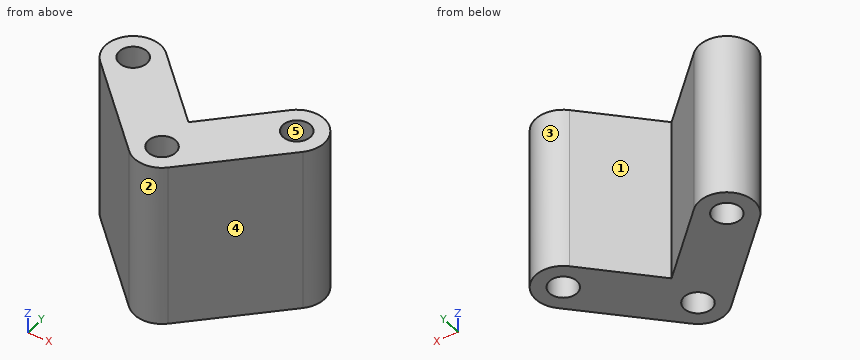
```python
from build123d import *

# Parameters (mm, degrees)
F0_R     = 12.5
F1_DEPTH = 150
F3_DEPTH = 50


# Not quite as in the source:
# - the program builds the solid bodies; features that only make, move or delete a surface that nothing else refers to are left out


with BuildPart() as f1:
    # F0 (on Top) → F1 (new body)
    with BuildSketch(Plane.XY):
        with BuildLine():
            Line((8.6845052377, -18.7444362128), (-50.6748429861, 39.3975202147))
            ThreePointArc((-50.6748429861, 39.3975202147), (-86.0282846169, 39.0312350068), (-85.661999409, 3.6777933759))
            Line((-85.661999409, 3.6777933759), (-9.0315715293, -71.3810327757))
            ThreePointArc((-9.0315715293, -71.3810327757), (8.4718011348, -78.5211674377), (25.9695737293, -71.3673200922))
            Line((25.9695737293, -71.3673200922), (98.7170861934, 0))
            ThreePointArc((98.7170861934, 0), (99.0182133881, 35.3918171352), (63.6258335307, 35.6173071466))
            Line((63.6258335307, 35.6173071466), (8.6845052377, -18.7444362128))
        make_face()
        with Locations((8.4620066821, -53.5211693563)):
            Circle(F0_R, mode=Mode.SUBTRACT)
        with Locations((-68.1684211975, 21.5376567953)):
            Circle(F0_R, mode=Mode.SUBTRACT)
        with Locations((81.2095191462, 17.8461507359)):
            Circle(F0_R, mode=Mode.SUBTRACT)
    extrude(amount=F1_DEPTH)

    # F0 (on Top) → F3 (join)
    with BuildSketch(Plane.XY):
        with BuildLine():
            Line((8.6845052377, -18.7444362128), (-50.6748429861, 39.3975202147))
            ThreePointArc((-50.6748429861, 39.3975202147), (-86.0282846169, 39.0312350068), (-85.661999409, 3.6777933759))
            Line((-85.661999409, 3.6777933759), (-9.0315715293, -71.3810327757))
            ThreePointArc((-9.0315715293, -71.3810327757), (8.4718011348, -78.5211674377), (25.9695737293, -71.3673200922))
            Line((25.9695737293, -71.3673200922), (98.7170861934, 0))
            ThreePointArc((98.7170861934, 0), (99.0182133881, 35.3918171352), (63.6258335307, 35.6173071466))
            Line((63.6258335307, 35.6173071466), (8.6845052377, -18.7444362128))
        make_face()
        with Locations((8.4620066821, -53.5211693563)):
            Circle(F0_R, mode=Mode.SUBTRACT)
        with Locations((-68.1684211975, 21.5376567953)):
            Circle(F0_R, mode=Mode.SUBTRACT)
        with Locations((81.2095191462, 17.8461507359)):
            Circle(F0_R, mode=Mode.SUBTRACT)
    extrude(amount=F3_DEPTH)


solid = f1.part
```
Verification items for the finished model (mm, model axes). Face numbers are marked on the shaded views. A direction names the side the tool comes from. Coordinates: 2 decimals unless noted, no trailing zeros. Loops run counter-clockwise (first coordinate to the right, second up) from the corner with the lowest first, then second, coordinate; pieces in that order, holes last. Notation, with made-up numbers: (70.5, -4.5) -> (122.5, -4.5) arc R31 cw to (122.5, 30.5) -> close; hole circle Ø11 at (0.25, 28). An arc over 180 degrees is marked (long way). Answer in a Markdown table with one row per item. Add a question column.
1. Depth check by flat-ended pin: P1, Ø8, axis at x = 10.5, z = 112.5, coming from the +Y side; P2, Ø1.5, axis at y = -53, z = 32.5, coming from the -X side; P3, Ø10, axis at x = 55.5, z = 16, coming from the +Y side. Enter the tip coordinate at first touch or a pass-through.
2. Section check B-B, the plane y = -61. Enter the section's corners in (x, z), then the cut area to 3 significant figures.
3. Material ranges on probe 1 along X at (y, z) = (-53, 89.5); probe 2 along X at (y, z) = (-64.5, 136); probe 3 along Y at (x, z) = (3.5, 105), recorded low to high. Write a range as [from, to].
4. Section check A-A, the plane x = 1. Enter the section's corners in (y, z), then the cut area to 3 significant figures.
5. Access from +Z, -Z, +X, -X, +Y, -Y to the whole of each face (thin tool, end or side, straight path). Record for the marked faces 1 and 2.
6. Section check C-C, the plane z = 103. Enter the section's corners in (x, y), then the cut area to 3 significant figures.
7. Draft check along Y on the marked faces 3, 4 and 5. Enter one of: +Y half, -Y half, draft (parallel to the pull), parting line (faces both ways), or undercut.
8. Section check D-D, the plane x = -27. Enter the section's corners in (y, z).
Derived:
| question | item | result |
|---|---|---|
| 1 | P1 | stops at y = -12.99 |
| 1 | P2 | stops at x = -28.56 |
| 1 | P3 | stops at y = 32.52 |
| 2 | outline | (-19.63, 0) -> (-1.55, 0) -> (-1.55, 150) -> (-19.63, 150) -> close; (18.48, 0) -> (36.54, 0) -> (36.54, 150) -> (18.48, 150) -> close |
| 2 | area | 5,420 mm² |
| 3 | probe 1 | x = [-27.8, -4.03], [20.95, 44.69] |
| 3 | probe 2 | x = [-16.06, 2.49], [14.44, 32.97] |
| 3 | probe 3 | y = [-78.02, -64.99], [-42.05, -13.67] |
| 4 | outline | (-77.38, 0) -> (-63.55, 0) -> (-63.55, 150) -> (-77.38, 150) -> close; (-43.49, 0) -> (-11.22, 0) -> (-11.22, 150) -> (-43.49, 150) -> close |
| 4 | area | 6,920 mm² |
| 5 | face 1 | +Z, -Z, +Y |
| 5 | face 2 | +Z, -Z, -Y |
| 6 | outline | (-85.66, 3.68) -> (-9.03, -71.38) arc R25 ccw to (25.97, -71.37) -> (98.72, 0) arc R25 ccw to (63.63, 35.62) -> (8.68, -18.74) -> (-50.67, 39.4) arc R25 ccw to start; hole circle Ø25 at (-68.17, 21.54); hole circle Ø25 at (8.46, -53.52); hole circle Ø25 at (81.21, 17.85) |
| 6 | area | 10,800 mm² |
| 7 | face 3 | parting line |
| 7 | face 4 | -Y half |
| 7 | face 5 | undercut |
| 8 | outline | (-53.78, 0) -> (16.21, 0) -> (16.21, 150) -> (-53.78, 150) -> close |
